from build123d import *

# Parameters (mm, degrees)
BOSS_EXTRUDE1_DEPTH = 1.25
SKETCH2_R           = 1.25
SKETCH2_W           = 2.5
SKETCH2_H           = 2.5
BOSS_EXTRUDE2_DEPTH = 6.5
CUT_EXTRUDE1_DEPTH  = 0.6


with BuildPart() as part:
    # Sketch1 → Boss-Extrude1 (new body)
    with BuildSketch(Plane(origin=(0, 0, 0), x_dir=(1, 0, 0), z_dir=(0, 1, 0))):
        Polygon((0, 0), (0, 80), (66.3, 80), (66.3, -15.623791318), align=None)
    extrude(amount=BOSS_EXTRUDE1_DEPTH)

    # Sketch2 → Boss-Extrude2 (add)
    with BuildSketch(Plane.XZ):
        with Locations(Location((56.5, 10.745914737, 0), (0, 0, 270))):
            Circle(SKETCH2_R)
        with Locations((56.5, -77.5)):
            Rectangle(SKETCH2_W, SKETCH2_H)
        with Locations((2.5, -25)):
            Rectangle(SKETCH2_W, SKETCH2_H)
    extrude(amount=-BOSS_EXTRUDE2_DEPTH)

    # Sketch4 → Cut-Extrude1 (cut)
    with BuildSketch(Plane(origin=(0, 1.25, 0), x_dir=(1, 0, 0), z_dir=(0, 1, 0))):
        Polygon((5, 75), (5, 3.958690319), (61.3, -9.308571388), (61.3, 75), align=None)
    extrude(amount=-CUT_EXTRUDE1_DEPTH, mode=Mode.SUBTRACT)


solid = part.part
The listing builds one solid part. Answer for the finished solid, in the listing's coordinates (mm). A direction names the side the tool comes from. Coordinates: 2 decimals unless noted, no trailing zeros. Order: outer loops, then holes, each group sorted by start corner. A loop starts at its lowest first (then second) coordinate and runs counter-clockwise, first axis right, second up. Notation, with made-up numbers: (-16, 18.25) -> (3, 18.25) arc R14 cw to (3, 23.25) -> close; hole circle Ø4 at (-36.75, 82.25). An arc over 180 degrees is marked (long way). Answer in a Markdown table with one row per item. Add a question column.
Item 1: Which of the six approach directions +Z, -Z, +X, -X, +Y, -Y give full straight-line access (tool end or side, diameter ignored) to faces 5 (the face through (2, 4, -26.25)), 6 (the face through (55.25, 4, -78)), 7 (the face through (3.75, 4, -25)), 8 (the face through (2, 4, -23.75)), 9 (the face through (33, 0.65, -33))?
Item 2: Find section C-C (x = 56.5). Write down the section's boundary in (y, z).
Item 3: Find section B-B (z = -39.5). Write down the section's boundary in (x, y), then the cut area to 3 significant figures.
Item 4: Determine the mould class of faces 1 (the face through (56, 4, -76.25)), 2 (the face through (57.74, 3.84, 10.91)), 3 (the face through (33.61, 0.62, 7.92)), 4 (the face through (57, 6.5, 11)) for opening direction Z: +Z half, -Z half, draft (parallel to the pull), parting line (faces both ways), or undercut.
Item 5: Find the intervals of material crossed by L1, parallel to X at y = 0.75, z = -40.5; L2, parallel to Y at x = 26.5, z = -67; L3, parallel to Y at x = 28.5, z = 5.5, in increasing order. Write a range as from..to.
Item 6: Each of these flat-tipped pins is pushed along its axis until it touches: P1, Ø2, axis at y = 5, z = -25, coming from the -X side; P2, Ø0.8, axis at y = 4.5, z = -24.5, coming from the +X side; P3, Ø1.5, axis at x = 58, y = 4.5, coming from the -Z side. Where does it stop, or does it pass through?
Item 7: Find section A-A (y = 5.5). Write down the section's boundary in (x, z).
Item 8: Find section D-D (x = 15). Write down the section's boundary in (y, z).
Result set:
| question | item | result |
|---|---|---|
| 1 | face 5 | -Z, +X, -X, +Y |
| 1 | face 6 | +Z, -Z, -X, +Y |
| 1 | face 7 | +Z, -Z, +X, +Y |
| 1 | face 8 | +Z, +X, -X, +Y |
| 1 | face 9 | +Y |
| 2 | outline | (0, -80) -> (1.25, -80) -> (1.25, -78.75) -> (6.5, -78.75) -> (6.5, -76.25) -> (1.25, -76.25) -> (1.25, -75) -> (0.65, -75) -> (0.65, 8.18) -> (1.25, 8.18) -> (1.25, 9.5) -> (6.5, 9.5) -> (6.5, 12) -> (1.25, 12) -> (1.25, 13.31) -> (0, 13.31) -> close |
| 3 | outline | (0, 0) -> (66.3, 0) -> (66.3, 1.25) -> (61.3, 1.25) -> (61.3, 0.65) -> (5, 0.65) -> (5, 1.25) -> (0, 1.25) -> close |
| 3 | area | 49.1 mm² |
| 4 | face 1 | undercut |
| 4 | face 2 | undercut |
| 4 | face 3 | +Z half |
| 4 | face 4 | draft |
| 5 | L1 | x = 0..5, 61.3..66.3 |
| 5 | L2 | y = 0..0.65 |
| 5 | L3 | y = 0..1.25 |
| 6 | P1 | stops at x = 1.25 |
| 6 | P2 | stops at x = 3.75 |
| 6 | P3 | stops at z = -78.75 |
| 7 | outline | (1.25, -26.25) -> (3.75, -26.25) -> (3.75, -23.75) -> (1.25, -23.75) -> close; (55.25, -78.75) -> (57.75, -78.75) -> (57.75, -76.25) -> (55.25, -76.25) -> close; circle Ø2.5 at (56.5, 10.75) |
| 8 | outline | (0, -80) -> (1.25, -80) -> (1.25, -75) -> (0.65, -75) -> (0.65, -1.6) -> (1.25, -1.6) -> (1.25, 3.53) -> (0, 3.53) -> close |
